The listing builds one solid part. Answer for the finished solid, in the listing's coordinates (mm). Face numbers are marked on the shaded views. A direction names the side the tool comes from. Give positions to 0.01 mm unless a question says otherwise; leave off trailing zeros. Loops run counter-clockwise (first coordinate to the right, second up) from the corner with the lowest first, then second, coordinate; pieces in that order, holes last.
Item 1: Each of these flat-tipped pins is pushed along its axis until it touches: pin 1 Ø3.5 at (y, z) = (18.76, -25.61) entering from +X; pin 2 Ø3 at (x, z) = (-24, -36.5) entering from +Y. Where does it stop, or does it pass through?
Item 2: Section C-C, the plane y = 33.5 is taken. Give the vertices of the cut face in (x, z), and give its area (3 significant figures).
Item 3: A tool of negligible diameter and unlimited length cuts with its end or side. For the marked faces 1 and 2, from which of +Z, -Z, +X, -X, +Y, -Y can it reach the whole face along a straight path? Write none if from no direction.
Item 4: Section A-A, the plane x = -21.25 is taken. Give the vertices of the cut face in (y, z).
Item 5: The mould has two halves that part along X. Classify the marked faces 3, 4 and 5: pulls with the +X half, pulls with the -X half, needs draft (parallel to the pull), parting line crosses it, or undercut.
Item 6: Section B-B, the plane x = -27.75 is taken. Give the vertices of the cut face in (y, z).
Item 7: Section D-D, the plane z = -26 is taken. Give the number of separate pieces and of enclosed holes in the cut face, and give its area (3 significant figures).
Item 8: Consider line 1 along X through (y, z) = (27.5, -42.75); line 2 along Y through (x, z) = (-14.25, -27.25); line 3 along Y through (x, z) = (-14.25, -24). Determine where each line is inside the solid, lowest interval first.
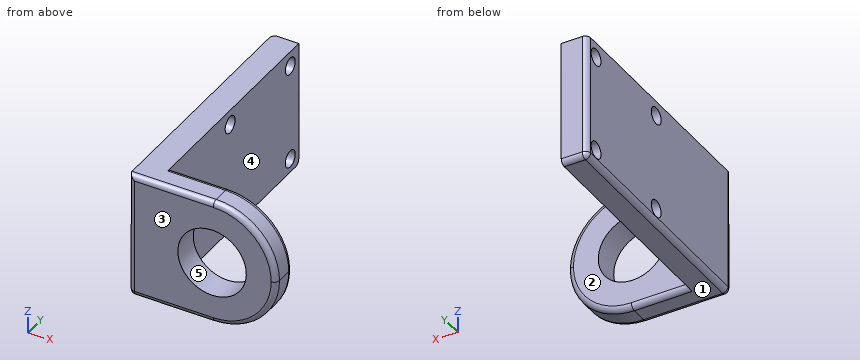
from build123d import *

# Parameters (mm, degrees)
CROQUIS1_W              = 24
CROQUIS1_H              = 46.5
CROQUIS1_R              = 1.6
SALIENTE_EXTRUIR1_DEPTH = 5
CROQUIS2_W              = 24
CROQUIS2_H              = 5
SALIENTE_EXTRUIR2_DEPTH = 23
CORTAR_EXTRUIR1_REACH   = 76.572
CROQUIS3_R              = 6.5
REDONDEO1_R             = 12
REDONDEO2_R             = 1
REDONDEO3_R             = 1


with BuildPart() as part:
    # Croquis1 → Saliente-Extruir1 (new body)
    with BuildSketch(Plane.ZY.offset(29.823119035)):
        with Locations((-34.755083615, 17.762616936)):
            Rectangle(CROQUIS1_W, CROQUIS1_H)
        with Locations((-44.105083615, 38.262616936)):
            Circle(CROQUIS1_R, mode=Mode.SUBTRACT)
        with Locations((-25.605083615, 38.262616936)):
            Circle(CROQUIS1_R, mode=Mode.SUBTRACT)
        with Locations((-25.605083615, 18.762616936)):
            Circle(CROQUIS1_R, mode=Mode.SUBTRACT)
        with Locations((-44.105083615, 18.762616936)):
            Circle(CROQUIS1_R, mode=Mode.SUBTRACT)
    extrude(amount=SALIENTE_EXTRUIR1_DEPTH)

    # Croquis2 → Saliente-Extruir2 (add)
    with BuildSketch(Plane(origin=(-29.823119035, 0, 0), x_dir=(0, 0, -1), z_dir=(1, 0, 0))):
        with Locations((34.755083615, -2.987383064)):
            Rectangle(CROQUIS2_W, CROQUIS2_H)
    extrude(amount=SALIENTE_EXTRUIR2_DEPTH)

    # Croquis3 → Cortar-Extruir1 (cut, up to next)
    with BuildSketch(Plane.XZ.offset(5.487383064), mode=Mode.PRIVATE) as cortar_extruir1_sk1:
        with Locations(Location((-19.047480384, -34.855083615, 0), (0, 0, 270))):
            Circle(CROQUIS3_R)
    cortar_extruir1_tool1 = extrude(cortar_extruir1_sk1.sketch, amount=-CORTAR_EXTRUIR1_REACH, mode=Mode.PRIVATE) & part.part
    add(cortar_extruir1_tool1.solids().sort_by_distance((-19.04748, -5.487383, -34.855084))[0], mode=Mode.SUBTRACT)

    # Redondeo1
    redondeo1_edges = [part.edges().sort_by_distance(p)[0] for p in [
        (-6.823119035, -2.987383064, -22.755083615),
        (-6.823119035, -2.987383064, -46.755083615),
    ]]
    fillet(redondeo1_edges, radius=REDONDEO1_R - 0.0001)  # a hair under: the kernel refuses the full size

    # Redondeo2
    redondeo2_edges = [part.edges().sort_by_distance(p)[0] for p in [
        (-26.823069035, -5.487383064, -22.755083615),
        (-10.337808371, -5.487383064, -26.269772952),
        (-10.337808371, -5.487383064, -43.240394279),
        (-24.323069035, -0.487383064, -22.755083615),
        (-10.337808371, -0.487383064, -26.269772952),
        (-10.337808371, -0.487383064, -43.240394279),
        (-34.823119035, -5.487383064, -34.755083615),
        (-34.823119035, 17.762616936, -46.755083615),
        (-26.823069035, -5.487383064, -46.755083615),
        (-24.323069035, -0.487383064, -46.755083615),
    ]]
    fillet(redondeo2_edges, radius=REDONDEO2_R)

    # Redondeo3
    redondeo3_edges = [part.edges().sort_by_distance(p)[0] for p in [
        (-31.823119035, 41.012616936, -46.755083615),
        (-34.823119035, 41.012616936, -34.255083615),
    ]]
    fillet(redondeo3_edges, radius=REDONDEO3_R)


solid = part.part
Worked answers:
1. pin 1: stops at x = -29.82
1. pin 2: stops at y = -0.49
2. outline: (-34.82, -45.76) arc R1 ccw to (-33.82, -46.76) - (-29.82, -46.76) - (-29.82, -22.76) - (-34.82, -22.76) - close
2. area: 120 mm2
3. face 1: -Z, +X, -X, +Y, -Y
3. face 2: +Z, -Z, +X, +Y
4. outline: (-5.49, -45.76) arc R1 ccw to (-4.49, -46.76) - (-1.49, -46.76) arc R1 ccw to (-0.49, -45.76) - (-0.49, -40.97) - (-5.49, -40.97) - close; (-5.49, -28.74) - (-0.49, -28.74) - (-0.49, -23.76) arc R1 ccw to (-1.49, -22.76) - (-4.49, -22.76) arc R1 ccw to (-5.49, -23.76) - close
5. face 3: needs draft
5. face 4: pulls with the +X half
5. face 5: undercut
6. outline: (-5.49, -45.76) arc R1 ccw to (-4.49, -46.76) - (-1.49, -46.76) arc R1 ccw to (-0.49, -45.76) - (-0.49, -23.76) arc R1 ccw to (-1.49, -22.76) - (-4.49, -22.76) arc R1 ccw to (-5.49, -23.76) - close
7. separate pieces: 3
7. enclosed holes: 0
7. area: 296 mm2
8. line 1: x = -34.82 to -29.82
8. line 2: y = -5.49 to -0.49
8. line 3: y = -5.21 to -0.76
